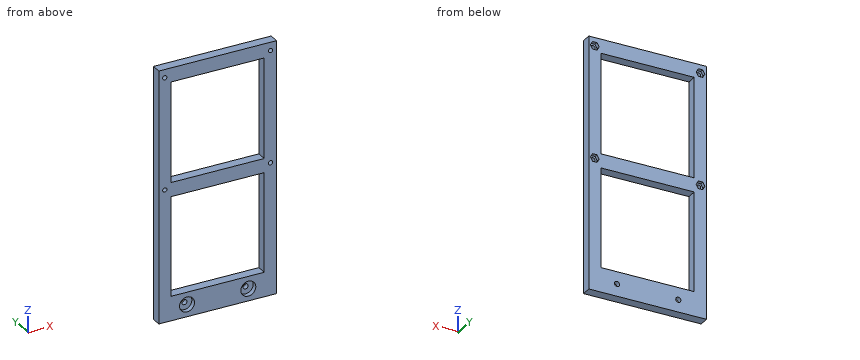
```python
from build123d import *

# Parameters (mm, degrees)
SKETCH_1_W               = 96
SKETCH_1_H               = 105
SKETCH_1_R               = 1.75
SKETCH_1_W_2             = 76
SKETCH_1_H_2             = 82
EXTRUDE_1_DEPTH          = 8
SKETCH_1_11_R            = 1.75
SKETCH_1_11_W            = 76
SKETCH_1_11_H            = 82
SKETCH_1_11_R_2          = 2.1
SKETCH_1_11_H_2          = 81.25
EXTRUDE_5_DEPTH          = 8
CUT_EXTRUDE_4_DEPTH      = 162.267053362
CUT_EXTRUDE_4_DEPTH_BACK = 162.267053362
SKETCH_1_12_W            = 76
SKETCH_1_12_H            = 81.25
SKETCH_3_R               = 6.1
CUT_EXTRUDE_5_DEPTH      = 4
CUT_EXTRUDE_6_DEPTH      = 3


with BuildPart() as part:
    # Эскиз1 → Бобышка-Вытянуть1 (new body)
    with BuildSketch(Plane(origin=(0, 0, 0), x_dir=(1, 0, 0), z_dir=(0, 1, 0))):
        Rectangle(SKETCH_1_W, SKETCH_1_H)
        with Locations(Location((-43.125, 45.75, 0), (0, 0, 270))):
            Circle(SKETCH_1_R, mode=Mode.SUBTRACT)
        with Locations(Location((43.125, 45.75, 0), (0, 0, 270))):
            Circle(SKETCH_1_R, mode=Mode.SUBTRACT)
        with Locations(Location((43.125, -45.75, 0), (0, 0, 270))):
            Circle(SKETCH_1_R, mode=Mode.SUBTRACT)
        with Locations(Location((-43.125, -45.75, 0), (0, 0, 270))):
            Circle(SKETCH_1_R, mode=Mode.SUBTRACT)
        Rectangle(SKETCH_1_W_2, SKETCH_1_H_2, mode=Mode.SUBTRACT)
    extrude(amount=EXTRUDE_1_DEPTH)

    # Эскиз1<11> → Бобышка-Вытянуть5 (add)
    # profile 1 of 3: a face of its own
    with BuildSketch(Plane(origin=(0, 0, 0), x_dir=(1, 0, 0), z_dir=(0, 1, 0))):
        Polygon((-48, -52.5), (48, -52.5), (48, 52.5), (38, 52.5), (-38, 52.5), (-48, 52.5), align=None)
        with Locations(Location((-43.125, -45.75, 0), (0, 0, 270))):
            Circle(SKETCH_1_11_R, mode=Mode.SUBTRACT)
        with Locations(Location((-43.125, 45.75, 0), (0, 0, 270))):
            Circle(SKETCH_1_11_R, mode=Mode.SUBTRACT)
        with Locations(Location((43.125, -45.75, 0), (0, 0, 270))):
            Circle(SKETCH_1_11_R, mode=Mode.SUBTRACT)
        Rectangle(SKETCH_1_11_W, SKETCH_1_11_H, mode=Mode.SUBTRACT)
        with Locations(Location((43.125, 45.75, 0), (0, 0, 270))):
            Circle(SKETCH_1_11_R, mode=Mode.SUBTRACT)
    # profile 2 of 3: a face of its own
    with BuildSketch(Plane(origin=(0, 0, 0), x_dir=(1, 0, 0), z_dir=(0, 1, 0))):
        Polygon((38, 52.5), (48, 52.5), (48, 153.75), (-48, 153.75), (-48, 52.5), (-38, 52.5), (-38, 133.75), (38, 133.75), align=None)
        with Locations(Location((-25, 143.75, 0), (0, 0, 270))):
            Circle(SKETCH_1_11_R_2, mode=Mode.SUBTRACT)
        with Locations(Location((25, 143.75, 0), (0, 0, 270))):
            Circle(SKETCH_1_11_R_2, mode=Mode.SUBTRACT)
    # profile 3 of 3: a face of its own
    with BuildSketch(Plane(origin=(0, 0, 0), x_dir=(1, 0, 0), z_dir=(0, 1, 0))):
        with Locations((0, 93.125)):
            Rectangle(SKETCH_1_11_W, SKETCH_1_11_H_2)
    extrude(amount=EXTRUDE_5_DEPTH)

    # Эскиз1<12> → Вырез-Вытянуть4 (cut, two sides: drawn at the far end of the back side and taken through both)
    with BuildSketch(Plane(origin=(0, 0, 0), x_dir=(1, 0, 0), z_dir=(0, 1, 0)).offset(-CUT_EXTRUDE_4_DEPTH_BACK)):
        with Locations((0, 93.125)):
            Rectangle(SKETCH_1_12_W, SKETCH_1_12_H)
    extrude(amount=CUT_EXTRUDE_4_DEPTH + CUT_EXTRUDE_4_DEPTH_BACK, mode=Mode.SUBTRACT)

    # Эскиз3 → Вырез-Вытянуть5 (cut)
    with BuildSketch(Plane.XZ):
        with Locations(Location((-25, -143.75, 0), (0, 0, 270))):
            Circle(SKETCH_3_R)
        with Locations(Location((25, -143.75, 0), (0, 0, 270))):
            Circle(SKETCH_3_R)
    extrude(amount=-CUT_EXTRUDE_5_DEPTH, mode=Mode.SUBTRACT)

    # Эскиз4 → Вырез-Вытянуть6 (cut)
    with BuildSketch(Plane(origin=(0, 8, 0), x_dir=(1, 0, 0), z_dir=(0, 1, 0))):
        Polygon((-39.545428331, 45.75), (-41.335214166, 48.85), (-44.914785834, 48.85), (-46.704571669, 45.75), (-44.914785834, 42.65), (-41.335214166, 42.65), align=None)
        Polygon((39.545428331, 45.75), (41.335214166, 42.65), (44.914785834, 42.65), (46.704571669, 45.75), (44.914785834, 48.85), (41.335214166, 48.85), align=None)
        Polygon((39.545428331, -45.75), (41.335214166, -48.85), (44.914785834, -48.85), (46.704571669, -45.75), (44.914785834, -42.65), (41.335214166, -42.65), align=None)
        Polygon((-39.545428331, -45.75), (-41.335214166, -42.65), (-44.914785834, -42.65), (-46.704571669, -45.75), (-44.914785834, -48.85), (-41.335214166, -48.85), align=None)
    extrude(amount=-CUT_EXTRUDE_6_DEPTH, mode=Mode.SUBTRACT)


solid = part.part
```
Part model, mm, in its own coordinate system. Give positions to 0.01 mm unless a question says otherwise; leave off trailing zeros. Order: outer loops, then holes, each group sorted by start corner. A loop starts at its lowest first (then second) coordinate and runs counter-clockwise, first axis right, second up. Notation, with made-up numbers: (2, 36.5) - (25, 36.5) arc R28 cw to (25, 59.5) - close; hole circle Ø10 at (29, 1.5). An arc over 180 degrees is marked (long way). Use one line per item in the form item = value.
Item 1: Probe probe 1 along X at (y, z) = (1.65, -45.75) (3 decimals); probe 2 along Z at (x, y) = (-22.5, 5.75); probe 3 along Z at (x, y) = (-25, 4.85). List the from-to ranges inside material, lowest first. Write a range as from..to.
Solution:
probe_1 = -48..-44.875, -41.375..41.375, 44.875..48
probe_2 = -153.75..-133.75, -52.5..-41, 41..52.5
probe_3 = -153.75..-145.85, -141.65..-133.75, -52.5..-41, 41..52.5
Item 2: Slice it at A-A on z = -64.5. Give the cut face in (x, y), and give its area (3 significant figures).
Solution:
outline = (-48, 0) - (-38, 0) - (-38, 8) - (-48, 8) - close; (38, 0) - (48, 0) - (48, 8) - (38, 8) - close
area = 160 mm2
Item 3: Slice it at C-C on z = -143.75. Give the cut face in (x, y).
Solution:
outline = (-48, 0) - (-31.1, 0) - (-31.1, 4) - (-27.1, 4) - (-27.1, 8) - (-48, 8) - close; (-22.9, 4) - (-18.9, 4) - (-18.9, 0) - (18.9, 0) - (18.9, 4) - (22.9, 4) - (22.9, 8) - (-22.9, 8) - close; (27.1, 4) - (31.1, 4) - (31.1, 0) - (48, 0) - (48, 8) - (27.1, 8) - close
Item 4: Pin check, flat tips, straight feed: pin 1 Ø4 at (x, z) = (-43.125, 45.75) entering from +Y; pin 2 Ø11 at (x, z) = (25, -143.75) entering from -Y. Stop position of each tip, or through.
Solution:
pin_1 = 5
pin_2 = 4
Item 5: Slice it at D-D on x = 25. Give the cut face in (y, z).
Solution:
outline = (0, -153.75) - (8, -153.75) - (8, -145.85) - (4, -145.85) - (4, -149.85) - (0, -149.85) - close; (0, -137.65) - (4, -137.65) - (4, -141.65) - (8, -141.65) - (8, -133.75) - (0, -133.75) - close; (0, -52.5) - (8, -52.5) - (8, -41) - (0, -41) - close; (0, 41) - (8, 41) - (8, 52.5) - (0, 52.5) - close
Item 6: Slice it at B-B on x = -12. Give the cut face in (y, z).
Solution:
outline = (0, -153.75) - (8, -153.75) - (8, -133.75) - (0, -133.75) - close; (0, -52.5) - (8, -52.5) - (8, -41) - (0, -41) - close; (0, 41) - (8, 41) - (8, 52.5) - (0, 52.5) - close
